Geometry: final body of the model. Coordinates: model frame, mm. A direction names the side the tool comes from. Round coordinates to 2 decimals unless told otherwise and drop trailing zeros. Write each loop counter-clockwise with the first axis right and the second up, starting at its lowest first coordinate (ties: lowest second). Pieces come first, ordered by that corner, then holes. Notation, with made-up numbers: M -29,60.5 L 4,60.5 A23 cw 4,68.5 Z; hole C 44,-4.75 d7. An arc over 180 degrees is marked long. Put each result on its own line as item: value. Start each with the question number.
```python
from build123d import *

# Parameters (mm, degrees)
EXTRUDE_1_REACH          = 32.84
EXTRUDE_1_END_RADIUS     = 17
SKETCH_4_W               = 16
SKETCH_4_H               = 20
SKETCH_7_R               = 1.6
EXTRUDE_2_DEPTH          = 8
FILLET_1_R               = 2
CUT_EXTRUDE_1_DEPTH      = 10
CUT_EXTRUDE_1_DEPTH_BACK = 28
SKETCH_9_W               = 16
SKETCH_9_H               = 20
EXTRUDE_3_DEPTH          = 4
FILLET_2_R               = 10


with BuildPart() as part:
    # 草图1 → 旋转1 (revolve)
    with BuildSketch(Plane.XY):
        with BuildLine():
            Line((0, 8.148347953), (0, 15.148347953))
            ThreePointArc((0, 15.148347953), (-9.649034823, 12.144637711), (-15.888316149, 4.194951128))
            ThreePointArc((-15.888316149, 4.194951128), (-15.414532258, 2.711018861), (-13.862245394, 2.841140494))
            ThreePointArc((-13.862245394, 2.841140494), (-8.835262424, 6.313648333), (-3, 8.124333536))
            Line((-3, 8.124333536), (-3, -5.851652047))
            Line((-3, -5.851652047), (0, -5.851652047))
            Line((0, -5.851652047), (0, 8.148347953))
        make_face()
    revolve(axis=Axis((0, 30.990444744, 0), (0, -1, 0)))

    # 凸台-拉伸1: up to this sphere (the profile starts outside it)
    extrude_1_end = Location((0, -1.851652047, 0)) * Sphere(EXTRUDE_1_END_RADIUS, mode=Mode.PRIVATE)
    # 草图4 → 凸台-拉伸1 (add, up to the surface)
    with BuildSketch(Plane(origin=(0, 15.148347953, 0), x_dir=(-1, 0, 0), z_dir=(0, -1, 0)), mode=Mode.PRIVATE) as extrude_1_sk1:
        Rectangle(SKETCH_4_W, SKETCH_4_H)
    extrude_1_tool1 = extrude(extrude_1_sk1.sketch, amount=EXTRUDE_1_REACH, mode=Mode.PRIVATE) - extrude_1_end
    add(extrude_1_tool1.solids().sort_by_distance((0, 15.148348, 0))[0])

    # 草图7 → 凸台-拉伸2 (add, symmetric)
    with BuildSketch(Plane(origin=(0, 0, 0), x_dir=(0, 0, -1), z_dir=(1, 0, 0))):
        Polygon((-10, 15.148347953), (-11.220970791, 35.111043921), (11.220970791, 35.111043921), (10, 15.148347953), align=None)
        with Locations((0, 29.148347953)):
            Circle(SKETCH_7_R, mode=Mode.SUBTRACT)
        with Locations((0, 19.148347953)):
            Circle(SKETCH_7_R, mode=Mode.SUBTRACT)
    extrude(amount=EXTRUDE_2_DEPTH, both=True)

    # 圆角1
    fillet_1_edges = [part.edges().sort_by_distance(p)[0] for p in [
        (3, 8.124333536, 0),
    ]]
    fillet(fillet_1_edges, radius=FILLET_1_R)

    # 草图8 → 切除-拉伸1 (cut, two sides: drawn at the far end of the back side and taken through both)
    with BuildSketch(Plane(origin=(8, 0, 0), x_dir=(0, 0, -1), z_dir=(1, 0, 0)).offset(-CUT_EXTRUDE_1_DEPTH_BACK)):
        Polygon((-10, 15.148347953), (10, 15.148347953), (22.074384404, 15.148347953), (22.074384404, -11.334225307), (-23.122772671, -11.334225307), (-23.122772671, 15.148347953), align=None)
    extrude(amount=CUT_EXTRUDE_1_DEPTH + CUT_EXTRUDE_1_DEPTH_BACK, mode=Mode.SUBTRACT)

    # 草图9 → 凸台-拉伸3 (add)
    with BuildSketch(Plane.XZ.offset(-15.148347953)):
        Rectangle(SKETCH_9_W, SKETCH_9_H)
    extrude(amount=EXTRUDE_3_DEPTH)

    # 圆角2
    # the kernel refuses this fillet: 10 mm, written as the material it adds along each edge
    with BuildSketch(Plane(origin=(8, 15.148347953, 10), x_dir=(0, 0.9981347984218685, 0.061048539534831796), z_dir=(-1, 0, 0)), Plane(origin=(-8, 15.148347953, -10), x_dir=(0, 0.9981347984218659, -0.06104853953487234), z_dir=(1, 0, 0))) as fillet_2_piece_1:
        with BuildLine():
            CenterArc((FILLET_2_R * 0.0305527632986, -FILLET_2_R), FILLET_2_R, 90, 3.5)
            Line((-FILLET_2_R * 0.0304957762363, -FILLET_2_R * 0.00186520157813), (0, 0))
            Line((0, 0), (FILLET_2_R * 0.0305527632986, 0))
        make_face()
    extrude(amount=16)


solid = part.part
```
1) First-contact query: pin 1 (6 mm diameter, centred on x = 6, y = 28.5, fed in from +Z); pin 2 (1.5 mm diameter, centred on x = -3, y = 19, fed in from -Z); pin 3 (4 mm diameter, centred on x = 3.5, y = 31, fed in from -Z). Flat tips, straight axial feed; report the tip coordinate or a pass-through.
2) Section B-B, the plane y = 28.5. Output: boundary loops of the cut face in (x, z), and give its area (3 significant figures).
3) Access query for faces 1 (the face through (0, 13, 10)), 2 (the face through (0, 13, -10)), 3 (the face through (0, 35.111, 0)). Directions: +Z, -Z, +X, -X, +Y, -Y. A direction counts if a zero-diameter tool reaches every point of the face in a straight line with its end or side. Return the directions, or none.
4) Draft query along Z for faces 4 (the face through (8, 23, -1)), 5 (the face through (-0.112, 27.586, 0.347)), 6 (the face through (0.11, 25.14, 10.61)), 7 (the face through (0.11, 25.42, -10.63)). Return one class per face: +Z half, -Z half, draft (parallel to the pull), parting line (faces both ways), or undercut.
5) Section A-A, the plane z = 0. Output: boundary loops of the cut face in (x, y), and give its area (3 significant figures).
6) Section C-C, the plane x = -5.75. Output: boundary loops of the cut face in (y, z).
7) Ray query, probe 1 along Y at (x, z) = (1.75, 0); probe 2 along Y at (x, z) = (3.5, 0.75); probe 3 along Z at (x, y) = (-6.75, 30). Return the intervals inside material, ascending.
8) Section D-D, the plane y = 14.5. Output: boundary loops of the cut face in (x, z), and give its area (3 significant figures).
Solved:
1. pin 1: stops at z = 11
1. pin 2: stops at z = -10.28
1. pin 3: stops at z = -11.09
2. outline: M -8,-10.82 L 8,-10.82 L 8,-1.46 L -8,-1.46 Z; M -8,1.46 L 8,1.46 L 8,10.82 L -8,10.82 Z
2. area: 299 mm2
3. face 1: +Z, +X, -X, -Y
3. face 2: -Z, +X, -X, -Y
3. face 3: +Z, -Z, +X, -X, +Y
4. face 4: draft
4. face 5: undercut
4. face 6: +Z half
4. face 7: -Z half
5. outline: M -8,11.15 L 8,11.15 L 8,17.55 L -8,17.55 Z; M -8,20.75 L 8,20.75 L 8,27.55 L -8,27.55 Z; M -8,30.75 L 8,30.75 L 8,35.11 L -8,35.11 Z
5. area: 281 mm2
6. outline: M 11.15,-10 L 14.84,-10 A10 cw 15.45,-10.02 L 35.11,-11.22 L 35.11,11.22 L 15.45,10.02 A10 cw 14.84,10 L 11.15,10 Z; hole C 19.15,0 d3.2; hole C 29.15,0 d3.2
7. probe 1: y = 11.15 to 17.55, 20.75 to 27.55, 30.75 to 35.11
7. probe 2: y = 11.15 to 17.74, 20.56 to 27.74, 30.56 to 35.11
7. probe 3: z = -10.91 to -1.35, 1.35 to 10.91
8. outline: M -8,-10 L 8,-10 L 8,10 L -8,10 Z
8. area: 320 mm2
